Design review of the part built by this model. Coordinates are the model's own, in mm. A direction names the side the tool comes from. Give positions to 0.01 mm unless a question says otherwise; leave off trailing zeros. Order: outer loops, then holes, each group sorted by start corner. A loop starts at its lowest first (then second) coordinate and runs counter-clockwise, first axis right, second up. Notation, with made-up numbers: M 23,46 L 70,46 A13 cw 70,70 Z; hole C 60,10 d2. An arc over 180 degrees is marked long. Answer as a JSON object with one key per item and string values.
from build123d import *

# Parameters (mm, degrees)
SKETCH_1_R      = 1.25
SKETCH_1_R_2    = 1.5
EXTRUDE_2_DEPTH = 3
EXTRUDE_3_DEPTH = 12
SKETCH_1_4_W    = 20.839933765
SKETCH_1_4_H    = 15
SKETCH_1_4_W_2  = 2
EXTRUDE_4_DEPTH = 1


with BuildPart() as part:
    # 草图1 → 凸台-拉伸2 (new body)
    with BuildSketch(Plane.XY):
        Polygon((-30.25, 31.520504216), (-30.25, 41.5), (-84.5, 41.5), (-84.5, -15), (-63.660066235, -15), (-63.660066235, -30), (-84.5, -30), (-84.5, -39.5), (60.5, -39.5), (60.5, 41.5), (30.25, 41.5), (30.25, 31.520504216), align=None)
        with Locations((-35, -25)):
            Circle(SKETCH_1_R, mode=Mode.SUBTRACT)
        with Locations((-28.75, -24.75)):
            Circle(SKETCH_1_R_2, mode=Mode.SUBTRACT)
        with Locations((28.75, -24.75)):
            Circle(SKETCH_1_R_2, mode=Mode.SUBTRACT)
        with Locations((35, -25)):
            Circle(SKETCH_1_R, mode=Mode.SUBTRACT)
        with Locations((-35, 25)):
            Circle(SKETCH_1_R, mode=Mode.SUBTRACT)
        with Locations((-28.75, 24.75)):
            Circle(SKETCH_1_R_2, mode=Mode.SUBTRACT)
        with Locations((28.75, 24.75)):
            Circle(SKETCH_1_R_2, mode=Mode.SUBTRACT)
        with Locations((35, 25)):
            Circle(SKETCH_1_R, mode=Mode.SUBTRACT)
    extrude(amount=-EXTRUDE_2_DEPTH)

    # 草图1<3> → 凸台-拉伸3 (add)
    with BuildSketch(Plane.XY):
        Polygon((-30.25, 43.5), (-86.5, 43.5), (-86.5, -15), (-84.5, -15), (-84.5, 41.5), (-30.25, 41.5), align=None)
        Polygon((62.5, 43.5), (30.25, 43.5), (30.25, 41.5), (60.5, 41.5), (60.5, -39.5), (-84.5, -39.5), (-84.5, -30), (-86.5, -30), (-86.5, -41.5), (62.5, -41.5), align=None)
    extrude(amount=-EXTRUDE_3_DEPTH)

    # 草图1<4> → 凸台-拉伸4 (add)
    with BuildSketch(Plane.XY):
        with Locations((-74.080033117, -22.5)):
            Rectangle(SKETCH_1_4_W, SKETCH_1_4_H)
        with Locations((-85.5, -22.5)):
            Rectangle(SKETCH_1_4_W_2, SKETCH_1_4_H)
    extrude(amount=-EXTRUDE_4_DEPTH)


solid = part.part
(1) Insertion check: pin 1 (12 mm diameter, centred on x = -69.5, y = -24, fed in from -Z); pin 2 (7 mm diameter, centred on x = 8.5, z = -7.5, fed in from +Y); pin 3 (2.5 mm diameter, centred on x = -6.5, z = -2, fed in from +Y). Each pin has a flat end and moves straight along its axis. Give the tip position at first contact, or say it passes through.
Checked values:
{"pin 1": "stops at z = -3", "pin 2": "stops at y = -39.5", "pin 3": "stops at y = 31.52"}
(2) We need section B-B (x = -28.75). Write out the cut boundary in (y, z).
Checked values:
{"outline": "M -41.5,-12 L -39.5,-12 L -39.5,-3 L -26.25,-3 L -26.25,0 L -41.5,0 Z; M -23.25,-3 L 23.25,-3 L 23.25,0 L -23.25,0 Z; M 26.25,-3 L 31.52,-3 L 31.52,0 L 26.25,0 Z"}
(3) Draft analysis for pull direction X (two halves, no side actions). For faces 1 (the flat face through (-86.5, 10, -6)), 2 (the flat face through (-77.7, -15, -2.8)), 3 (the flat face through (-58, 41.5, -7)), 4 (the flat face through (-84.5, 13, -7)), state which applies: +X half, -X half, draft (parallel to the pull), parting line (faces both ways), or undercut.
Checked values:
{"face 1": "-X half", "face 2": "draft", "face 3": "undercut", "face 4": "undercut"}
(4) Tool access review of faces 5 (the flat face through (-13, -41.5, -6)), 6 (the flat face through (-75, -22, -1)), 7 (the flat face through (0, 31.521, -1)), 8 (the flat face through (60.5, 2, -7)): name each direction out of +Z, -Z, +X, -X, +Y, -Y from which nothing blocks a thin tool from reaching the whole face with its end or side.
Checked values:
{"face 5": "+Z, -Z, +X, -X, -Y", "face 6": "-Z, -X", "face 7": "+Z, -Z, +Y", "face 8": "-Z"}
(5) To check wall thickness, follow L1, parallel to Y at x = -28.75, z = -1.8; L2, parallel to Y at x = -35, z = -1.5; L3, parallel to X at y = 36.5, z = -11.25. State the ranges of each line that lie inside material, in increasing order. Write a range as from..to.
Checked values:
{"L1": "y = -41.5..-26.25, -23.25..23.25, 26.25..31.52", "L2": "y = -41.5..-26.25, -23.75..23.75, 26.25..43.5", "L3": "x = -86.5..-84.5, 60.5..62.5"}
(6) We need section C-C (x = -61). Write out the cut boundary in (y, z), plus the area to 3 significant figures.
Checked values:
{"outline": "M -41.5,-12 L -39.5,-12 L -39.5,-3 L 41.5,-3 L 41.5,-12 L 43.5,-12 L 43.5,0 L -41.5,0 Z", "area": "291 mm^2"}
(7) We need section D-D (y = 12.5). Write out the cut boundary in (x, z).
Checked values:
{"outline": "M -86.5,-12 L -84.5,-12 L -84.5,-3 L 60.5,-3 L 60.5,-12 L 62.5,-12 L 62.5,0 L -86.5,0 Z"}
(8) We need section A-A (z = -8.75). Write out the cut boundary in (x, y).
Checked values:
{"outline": "M -86.5,-41.5 L 62.5,-41.5 L 62.5,43.5 L 30.25,43.5 L 30.25,41.5 L 60.5,41.5 L 60.5,-39.5 L -84.5,-39.5 L -84.5,-30 L -86.5,-30 Z; M -86.5,-15 L -84.5,-15 L -84.5,41.5 L -30.25,41.5 L -30.25,43.5 L -86.5,43.5 Z"}
